Check sheet for the modelled part. Datum: model origin and axes. Units: mm. A direction names the side the tool comes from. Give positions to 0.01 mm unless a question says otherwise; leave off trailing zeros. Loops run counter-clockwise (first coordinate to the right, second up) from the corner with the lowest first, then second, coordinate; pieces in that order, holes last. Notation, with made-up numbers: (77.5, 69.5) - (88.5, 69.5) arc R20 ccw to (88.5, 73.5) - close; hole circle Ø1 at (36.25, 54). An arc over 180 degrees is marked (long way). Use CSV: the item, a comma, the result in double quotes.
from build123d import *

# Parameters (mm, degrees)
BOSS_EXTRUDE2_DEPTH   = 4
SKETCH1_W             = 4.0000000000000036
SKETCH1_H             = 29.19999999999999
BOSS_EXTRUDE2_2_DEPTH = 4
BOSS_EXTRUDE2_3_DEPTH = 4
BOSS_EXTRUDE2_4_DEPTH = 4
SKETCH1_W_2           = 4
SKETCH1_H_2           = 17.435500273431558
BOSS_EXTRUDE2_5_DEPTH = 4
BOSS_EXTRUDE2_6_DEPTH = 4
BOSS_EXTRUDE2_7_DEPTH = 4
SKETCH1_H_3           = 17.43550027343155
BOSS_EXTRUDE2_8_DEPTH = 4
CUT_EXTRUDE1_DEPTH    = 4
SKETCH3_W             = 162.8
SKETCH3_H             = 200.6710005468631
BOSS_EXTRUDE3_DEPTH   = 40
SKETCH4_W             = 162.8
SKETCH4_H             = 200.6710005468631
BOSS_EXTRUDE4_DEPTH   = 4
FILLET1_R             = 5
FILLET2_R             = 5
FILLET3_R             = 5
FILLET4_R             = 5
SKETCH5_R             = 1.9999999999999967
SKETCH5_R_2           = 2
SKETCH5_R_3           = 2.0000000000000036
CUT_EXTRUDE2_DEPTH    = 4
BOSS_EXTRUDE5_DEPTH   = 8
SKETCH7_R             = 2.0000000000000036
CUT_EXTRUDE3_DEPTH    = 8
SKETCH8_W             = 16
SKETCH8_H             = 12
BOSS_EXTRUDE6_DEPTH   = 8
SKETCH9_R             = 1.9999999999999967
CUT_EXTRUDE4_DEPTH    = 8
SKETCH11_R            = 2
SKETCH11_R_2          = 1.9999999999999967
CUT_EXTRUDE5_DEPTH    = 8
SKETCH12_W            = 15.199999999999989
SKETCH12_H            = 20.419999999999987
CUT_EXTRUDE6_DEPTH    = 4
BOSS_EXTRUDE7_DEPTH   = 44
SKETCH14_W            = 24.419999999999987
SKETCH14_H            = 15.199999999999989
BOSS_EXTRUDE8_DEPTH   = 19.58
CHAMFER2_SIZE2        = 24.42
CHAMFER2_SIZE         = 28.42


with BuildPart() as part:
    # Sketch1 → Boss-Extrude2 (new body)
    with BuildSketch(Plane(origin=(0, 95.46497129757712, 0), x_dir=(1, 0, 0), z_dir=(0, 1, 0))):
        Polygon((5.580685050864992, -64.97044696543385), (5.580685050864992, -47.5349466920023), (1.580685050864986, -47.5349466920023), (1.5806850508649888, -64.97044696543384), align=None)
    extrude(amount=-BOSS_EXTRUDE2_DEPTH)



with BuildPart() as body_2:
    # Sketch1 → Boss-Extrude2 2 (new body)
    with BuildSketch(Plane(origin=(0, 95.46497129757712, 0), x_dir=(1, 0, 0), z_dir=(0, 1, 0))):
        with Locations((3.5806850508649903, -115.37044696543384)):
            Rectangle(SKETCH1_W, SKETCH1_H)
    extrude(amount=-BOSS_EXTRUDE2_2_DEPTH)


with BuildPart() as body_3:
    # Sketch1 → Boss-Extrude2 3 (new body)
    with BuildSketch(Plane(origin=(0, 95.46497129757712, 0), x_dir=(1, 0, 0), z_dir=(0, 1, 0))):
        Polygon((5.580685050864992, -165.77044696543385), (1.5806850508649957, -165.77044696543385), (1.5806850508649888, -194.97044696543384), (5.580685050864992, -194.97044696543384), align=None)
    extrude(amount=-BOSS_EXTRUDE2_3_DEPTH)


with BuildPart() as body_4:
    # Sketch1 → Boss-Extrude2 4 (new body)
    with BuildSketch(Plane(origin=(0, 95.46497129757712, 0), x_dir=(1, 0, 0), z_dir=(0, 1, 0))):
        Polygon((5.580685050864992, -230.77044696543385), (1.5806850508649888, -230.77044696543385), (1.5806850508649888, -248.2059472388654), (5.580685050864986, -248.2059472388654), align=None)
    extrude(amount=-BOSS_EXTRUDE2_4_DEPTH)


with BuildPart() as body_5:
    # Sketch1 → Boss-Extrude2 5 (new body)
    with BuildSketch(Plane(origin=(0, 95.46497129757712, 0), x_dir=(1, 0, 0), z_dir=(0, 1, 0))):
        with Locations((162.380685050865, -239.48819710214963)):
            Rectangle(SKETCH1_W_2, SKETCH1_H_2)
    extrude(amount=-BOSS_EXTRUDE2_5_DEPTH)


with BuildPart() as body_6:
    # Sketch1 → Boss-Extrude2 6 (new body)
    with BuildSketch(Plane(origin=(0, 95.46497129757712, 0), x_dir=(1, 0, 0), z_dir=(0, 1, 0))):
        with Locations((162.380685050865, -180.37044696543384)):
            Rectangle(SKETCH1_W_2, SKETCH1_H)
    extrude(amount=-BOSS_EXTRUDE2_6_DEPTH)


with BuildPart() as body_7:
    # Sketch1 → Boss-Extrude2 7 (new body)
    with BuildSketch(Plane(origin=(0, 95.46497129757712, 0), x_dir=(1, 0, 0), z_dir=(0, 1, 0))):
        Polygon((164.380685050865, -148.66643660097685), (164.380685050865, -100.77044696543385), (160.380685050865, -100.77044696543385), (160.380685050865, -123.46643660097686), (136.36222349016015, -123.46643660097686), (136.36222349016015, -138.66643660097685), (160.380685050865, -138.66643660097685), (160.380685050865, -148.66643660097685), align=None)
    extrude(amount=-BOSS_EXTRUDE2_7_DEPTH)

    # Sketch2 → Cut-Extrude1 (cut)
    with BuildSketch(Plane(origin=(0, 95.46497129757712, 0), x_dir=(1, 0, 0), z_dir=(0, 1, 0))):
        Polygon((160.380685050865, -123.46643660097686), (136.36222349016015, -123.46643660097686), (136.36222349016015, -138.66643660097685), (160.380685050865, -138.66643660097685), (164.380685050865, -138.66643660097685), (164.380685050865, -123.46643660097686), align=None)
    extrude(amount=-CUT_EXTRUDE1_DEPTH, mode=Mode.SUBTRACT)


with BuildPart() as body_8:
    # Sketch1 → Boss-Extrude2 8 (new body)
    with BuildSketch(Plane(origin=(0, 95.46497129757712, 0), x_dir=(1, 0, 0), z_dir=(0, 1, 0))):
        with Locations((162.380685050865, -56.25269682871807)):
            Rectangle(SKETCH1_W_2, SKETCH1_H_3)
    extrude(amount=-BOSS_EXTRUDE2_8_DEPTH)


with BuildPart() as cut_extrude1_piece_1:
    # of the separate pieces the step leaves, piece 1, a body of its own (cut_extrude1_pieces)
    add(body_7.part.solids().sort_by_distance((164.380685051, 95.464971298, 123.466436601))[0])


with BuildPart() as cut_extrude1_piece_2:
    # of the separate pieces the step leaves, piece 2, a body of its own (cut_extrude1_pieces)
    add(body_7.part.solids().sort_by_distance((164.380685051, 95.464971298, 148.666436601))[0])


with BuildPart() as part_1:
    add(part.part)

    add(body_2.part)  # Boss-Extrude3 merges body 2

    add(body_3.part)  # Boss-Extrude3 merges body 3

    add(body_4.part)  # Boss-Extrude3 merges body 4

    add(body_5.part)  # Boss-Extrude3 merges body 5

    add(body_6.part)  # Boss-Extrude3 merges body 6

    add(body_8.part)  # Boss-Extrude3 merges body 8

    add(cut_extrude1_piece_1.part)  # Boss-Extrude3 merges Cut-Extrude1 piece 1

    add(cut_extrude1_piece_2.part)  # Boss-Extrude3 merges Cut-Extrude1 piece 2
    # Sketch3 → Boss-Extrude3 (add)
    with BuildSketch(Plane.XZ.offset(-91.46497129757712)):
        with Locations((82.98068505086499, 147.87044696543384)):
            Rectangle(SKETCH3_W, SKETCH3_H)
        Polygon((160.380685050865, 51.5349466920023), (160.380685050865, 244.2059472388654), (5.580685050864989, 244.2059472388654), (5.580685050864981, 51.5349466920023), align=None, mode=Mode.SUBTRACT)
    extrude(amount=BOSS_EXTRUDE3_DEPTH)

    # Sketch4 → Boss-Extrude4 (add)
    with BuildSketch(Plane.XZ.offset(-51.46497129757712)):
        with Locations((82.98068505086499, 147.87044696543384)):
            Rectangle(SKETCH4_W, SKETCH4_H)
    extrude(amount=BOSS_EXTRUDE4_DEPTH)

    # Fillet1
    fillet1_edges = [part_1.edges().sort_by_distance(p)[0] for p in [
        (1.5806850508649881, 71.46497129757712, 248.2059472388654),
    ]]
    fillet(fillet1_edges, radius=FILLET1_R)

    # Fillet2
    fillet2_edges = [part_1.edges().sort_by_distance(p)[0] for p in [
        (164.380685050865, 71.46497129757712, 248.2059472388654),
    ]]
    fillet(fillet2_edges, radius=FILLET2_R)

    # Fillet3
    fillet3_edges = [part_1.edges().sort_by_distance(p)[0] for p in [
        (164.380685050865, 71.46497129757712, 47.53494669200231),
    ]]
    fillet(fillet3_edges, radius=FILLET3_R)

    # Fillet4
    fillet4_edges = [part_1.edges().sort_by_distance(p)[0] for p in [
        (1.5806850508649881, 71.46497129757712, 47.53494669200231),
    ]]
    fillet(fillet4_edges, radius=FILLET4_R)

    # Sketch5 → Cut-Extrude2 (cut)
    with BuildSketch(Plane.XZ.offset(-47.46497129757712)):
        with Locations(Location((149.380685050865, 62.53494669200229, 0), (0, 0, 270))):
            Circle(SKETCH5_R)
        with Locations(Location((16.580685050864986, 62.53494669200231, 0), (0, 0, 270))):
            Circle(SKETCH5_R_2)
        with Locations(Location((149.380685050865, 233.20594723886538, 0), (0, 0, 270))):
            Circle(SKETCH5_R)
        with Locations(Location((16.58068505086499, 233.2059472388654, 0), (0, 0, 270))):
            Circle(SKETCH5_R_3)
    extrude(amount=-CUT_EXTRUDE2_DEPTH, mode=Mode.SUBTRACT)

    # Sketch6 → Boss-Extrude5 (add)
    with BuildSketch(Plane(origin=(0, 91.46497129757712, 0), x_dir=(1, 0, 0), z_dir=(0, 1, 0))):
        Polygon((21.580685050864982, -63.534946692002315), (21.580685050864975, -51.5349466920023), (5.580685050864992, -51.5349466920023), (5.580685050864982, -63.53494669200232), align=None)
    boss_extrude5 = extrude(amount=-BOSS_EXTRUDE5_DEPTH)

    # Sketch7 → Cut-Extrude3 (cut)
    with BuildSketch(Plane(origin=(0, 91.46497129757712, 0), x_dir=(1, 0, 0), z_dir=(0, 1, 0))):
        with Locations(Location((15.980685050864993, -57.934946692002306, 0), (0, 0, 270))):
            Circle(SKETCH7_R)
    cut_extrude3 = extrude(amount=-CUT_EXTRUDE3_DEPTH, mode=Mode.SUBTRACT)

    # Mirror1: Boss-Extrude5, Cut-Extrude3 across plane
    add(boss_extrude5.mirror(Plane.ZY.offset(-82.980685050865)))
    add(cut_extrude3.mirror(Plane.ZY.offset(-82.980685050865)), mode=Mode.SUBTRACT)

    # Sketch8 → Boss-Extrude6 (add)
    with BuildSketch(Plane(origin=(0, 91.46497129757712, 0), x_dir=(1, 0, 0), z_dir=(0, 1, 0))):
        with Locations((152.380685050865, -238.2059472388654)):
            Rectangle(SKETCH8_W, SKETCH8_H)
    extrude(amount=-BOSS_EXTRUDE6_DEPTH)

    # Sketch9 → Cut-Extrude4 (cut)
    with BuildSketch(Plane(origin=(0, 91.46497129757712, 0), x_dir=(1, 0, 0), z_dir=(0, 1, 0))):
        with Locations(Location((149.98068505086505, -237.8059472388654, 0), (0, 0, 270))):
            Circle(SKETCH9_R)
    extrude(amount=-CUT_EXTRUDE4_DEPTH, mode=Mode.SUBTRACT)

    # Sketch11 → Cut-Extrude5 (cut)
    with BuildSketch(Plane(origin=(0, 91.46497129757712, 0), x_dir=(1, 0, 0), z_dir=(0, 1, 0))):
        with Locations((11.180685050864989, -243.87594723886542)):
            Circle(SKETCH11_R)
        with Locations((74.680685050865, -243.87594723886542)):
            Circle(SKETCH11_R_2)
    extrude(amount=-CUT_EXTRUDE5_DEPTH, mode=Mode.SUBTRACT)

    # Sketch12 → Cut-Extrude6 (cut)
    with BuildSketch(Plane(origin=(164.380685050865, 0, 0), x_dir=(0, 0, -1), z_dir=(1, 0, 0))):
        with Locations((-131.06643660097686, 81.25497129757713)):
            Rectangle(SKETCH12_W, SKETCH12_H)
    extrude(amount=-CUT_EXTRUDE6_DEPTH, mode=Mode.SUBTRACT)

    # Sketch13 → Boss-Extrude7 (add)
    with BuildSketch(Plane(origin=(0, 51.46497129757712, 0), x_dir=(1, 0, 0), z_dir=(0, 1, 0))):
        Polygon((135.960685050865, -123.46643660097686), (160.380685050865, -123.46643660097686), (160.380685050865, -120.46643660097686), (132.960685050865, -120.46643660097686), (132.960685050865, -141.66643660097685), (160.380685050865, -141.66643660097685), (160.380685050865, -138.66643660097685), (135.960685050865, -138.66643660097685), align=None)
    extrude(amount=BOSS_EXTRUDE7_DEPTH)

    # Sketch14 → Boss-Extrude8 (add)
    with BuildSketch(Plane(origin=(0, 51.46497129757712, 0), x_dir=(1, 0, 0), z_dir=(0, 1, 0))):
        with Locations((148.17068505086502, -131.06643660097686)):
            Rectangle(SKETCH14_W, SKETCH14_H)
    extrude(amount=BOSS_EXTRUDE8_DEPTH)

    # Chamfer2
    chamfer2_edges = [part_1.edges().sort_by_distance(p)[0] for p in [
        (135.960685050865, 71.04497129757712, 131.06643660097686),
    ]]
    chamfer2_side = [part_1.faces().sort_by_distance(p)[0] for p in [
        (136.44908505086502, 71.04497129757712, 131.06643660097686),
    ]]
    chamfer(chamfer2_edges, length=CHAMFER2_SIZE - 0.0001, length2=CHAMFER2_SIZE2 - 0.0001, reference=chamfer2_side[0])  # a hair under: the kernel refuses the full size


solid = part_1.part
1. Scan lines: line 1 along Z through (x, y) = (154, 64); line 2 along Z through (x, y) = (77, 87); line 3 along X through (y, z) = (70, 168). Record each from-to range of solid material in increasing order.
Completed:
line 1,"z = 47.53 to 51.53, 120.47 to 141.67, 244.21 to 248.21"
line 2,"z = 47.53 to 51.53, 244.21 to 248.21"
line 3,"x = 1.58 to 5.58, 160.38 to 164.38"
2. Set-up check for faces 1 (the face through (162, 91.465, 157)), 2 (the face through (82, 72, 51.535)), 3 (the face through (132.961, 73, 131)): record each of +Z, -Z, +X, -X, +Y, -Y from which the full face is reachable in a straight line by a thin tool's end or side.
Completed:
face 1,"+X, -X, +Y"
face 2,"none"
face 3,"+Y"
3. Sectioned sample at B-B, the plane y = 63. Record the boundary of the cut face in (x, z).
Completed:
outline,"(1.58, 52.53) arc R5 ccw to (6.58, 47.53) - (159.38, 47.53) arc R5 ccw to (164.38, 52.53) - (164.38, 243.21) arc R5 ccw to (159.38, 248.21) - (6.58, 248.21) arc R5 ccw to (1.58, 243.21) - close; hole (5.58, 51.53) - (160.38, 51.53) - (160.38, 120.47) - (132.96, 120.47) - (132.96, 141.67) - (160.38, 141.67) - (160.38, 244.21) - (5.58, 244.21) - close"
4. Sectioned sample at A-A, the plane z = 94. Record the boundary of the cut face in (x, y).
Completed:
outline,"(1.58, 47.46) - (164.38, 47.46) - (164.38, 91.46) - (160.38, 91.46) - (160.38, 51.46) - (5.58, 51.46) - (5.58, 91.46) - (1.58, 91.46) - close"
5. Sectioned sample at D-D, the plane y = 88. State how many separate pieces and enclosed holes the cut face has, and give its area (3 significant figures).
Completed:
separate pieces,"1"
enclosed holes,"4"
area,"3,630 mm²"
6. Go/stop test with flat-tipped pins: pin 1 Ø1.5 at (y, z) = (76.5, 133.5) entering from +X; pin 2 Ø5 at (x, z) = (149.38, 233.21) entering from +Y (3 decimals); pin 3 Ø3 at (x, y) = (4, 93.5) entering from -Z. Record where each tip stops, or that it passes through.
Completed:
pin 1,"stops at x = 158.9"
pin 2,"stops at y = 91.465"
pin 3,"stops at z = 47.65"
7. Release check for a two-part mould opening along X. For faces 4 (the face through (164.381, 72, 147)), 5 (the face through (162, 93, 100.77)), 6 (the face through (17.93, 49.44, 64.01)) record: released by +X, released by -X, zero draft, split by the parting line, or undercut.
Completed:
face 4,"released by +X"
face 5,"zero draft"
face 6,"undercut"
8. Sectioned sample at C-C, the plane x = 90. Record the boundary of the cut face in (y, z), and give its area (3 significant figures).
Completed:
outline,"(47.46, 47.53) - (91.46, 47.53) - (91.46, 51.53) - (51.46, 51.53) - (51.46, 244.21) - (91.46, 244.21) - (91.46, 248.21) - (47.46, 248.21) - close"
area,"1,120 mm²"
